from build123d import *
from build123d.topology import SkipClean

# Parameters (mm, degrees)
SKETCH_1_R          = 4
EXTRUDE_1_DEPTH     = 12
SKETCH_3_R          = 15
EXTRUDE_3_DEPTH     = 25
CUT_EXTRUDE_START   = -5
CUT_EXTRUDE_2_DEPTH = 5
SKETCH_6_R          = 4
SKETCH_6_W          = 8
SKETCH_6_H          = 5
CUT_EXTRUDE_3_DEPTH = 69.629439747
SKETCH_10_R         = 7.5
CUT_EXTRUDE_4_DEPTH = 68.037303048


with BuildPart() as part:
    # Sketch 1 → Extrude 1 (new body)
    with BuildSketch(Plane(origin=(0, 0, 0), x_dir=(1, 0, 0), z_dir=(0, 1, 0))):
        with BuildLine():
            ThreePointArc((-40, 25), (-47.071067812, 22.071067812), (-50, 15))
            Line((-50, 15), (-50, -15))
            ThreePointArc((-50, -15), (-47.071067812, -22.071067812), (-40, -25))
            Line((-40, -25), (40, -25))
            ThreePointArc((40, -25), (47.071067812, -22.071067812), (50, -15))
            Line((50, -15), (50, 15))
            ThreePointArc((50, 15), (47.071067812, 22.071067812), (40, 25))
            Line((40, 25), (-40, 25))
        make_face()
        with Locations(Location((-40, -15, 0), (0, 0, 270))):
            Circle(SKETCH_1_R, mode=Mode.SUBTRACT)
        with Locations(Location((40, -15, 0), (0, 0, 270))):
            Circle(SKETCH_1_R, mode=Mode.SUBTRACT)
        with Locations(Location((-40, 15, 0), (0, 0, 270))):
            Circle(SKETCH_1_R, mode=Mode.SUBTRACT)
        with Locations(Location((40, 15, 0), (0, 0, 270))):
            Circle(SKETCH_1_R, mode=Mode.SUBTRACT)
    extrude(amount=EXTRUDE_1_DEPTH)

    # Sketch 3 → Extrude 3 (add)
    with BuildSketch(Plane(origin=(0, 12, 0), x_dir=(1, 0, 0), z_dir=(0, 1, 0))):
        Circle(SKETCH_3_R)
        with BuildLine():
            Line((-50, -4), (-14.456832295, -4))
            ThreePointArc((-14.456832295, -4), (-15, 0), (-14.456832295, 4))
            Line((-14.456832295, 4), (-50, 4))
            Line((-50, 4), (-50, -4))
        make_face()
    extrude_3 = extrude(amount=EXTRUDE_3_DEPTH)

    # Sketch 7 → Cut-Extrude 2 (cut)
    with BuildSketch(Plane(origin=(0, 37, 0), x_dir=(1, 0, 0), z_dir=(0, 1, 0)).offset(CUT_EXTRUDE_START)):
        with BuildLine():
            Line((-14.456832295, 4), (-50, 4))
            Line((-50, 4), (-50, -4))
            Line((-50, -4), (-14.456832295, -4))
            ThreePointArc((-14.456832295, -4), (-15, 0), (-14.456832295, 4))
        make_face()
    cut_extrude_2 = extrude(amount=CUT_EXTRUDE_2_DEPTH, mode=Mode.SUBTRACT)

    # Sketch 6 → Cut-Extrude 3 (cut, symmetric)
    with BuildSketch(Plane.XY.offset(4)):
        with Locations((0.161482291, 22)):
            Circle(SKETCH_6_R)
        Polygon((-14.456832295, 32), (-50, 12), (-50, 32), align=None)
        with Locations((0.271583853, 34.5)):
            Rectangle(SKETCH_6_W, SKETCH_6_H)
    cut_extrude_3 = extrude(amount=CUT_EXTRUDE_3_DEPTH, both=True, mode=Mode.SUBTRACT)

    # Mirror 3: Extrude 3, Cut-Extrude 2, Cut-Extrude 3 across plane
    with SkipClean():  # the faces are left unmerged after this step: merging them gives an invalid solid
        add(extrude_3.mirror(Plane(origin=(0, 0, 0), x_dir=(0, 0, 1), z_dir=(1, 0, 0))))
        add(cut_extrude_2.mirror(Plane(origin=(0, 0, 0), x_dir=(0, 0, 1), z_dir=(1, 0, 0))), mode=Mode.SUBTRACT)
        add(cut_extrude_3.mirror(Plane(origin=(0, 0, 0), x_dir=(0, 0, 1), z_dir=(1, 0, 0))), mode=Mode.SUBTRACT)
    add(part.part.scale(1), mode=Mode.REPLACE)  # the faces are merged on a copy

    # Sketch 10 → Cut-Extrude 4 (cut, through all)
    with BuildSketch(Plane(origin=(0, 37, 0), x_dir=(1, 0, 0), z_dir=(0, 1, 0))):
        with Locations(Location((0, 0, 0), (0, 0, 270))):
            Circle(SKETCH_10_R)
    extrude(amount=-CUT_EXTRUDE_4_DEPTH, mode=Mode.SUBTRACT)


solid = part.part
Read the model definition and answer for the solid it produces. Units are mm, in the model's axes. A direction names the side the tool comes from. Round coordinates to 2 decimals unless told otherwise and drop trailing zeros. Write each loop counter-clockwise with the first axis right and the second up, starting at its lowest first coordinate (ties: lowest second). Pieces come first, ordered by that corner, then holes. Notation, with made-up numbers: (7.25, -14) - (36.25, -14) arc R32 ccw to (36.25, 16) - close; hole circle Ø1 at (-17.75, 52). An arc over 180 degrees is marked (long way). One line per question, with ' | ' between items. Start each with the question number.
1. Section A-A (z = 0) is taken. Determine the outline of the cut face in (x, y).
2. For a pull along X with two mould halves and no side action, classify faces 1 (the face through (31.98, 22.14, -0.06)), 2 (the face through (-12, 0, 0)), 3 (the face through (-50, 6, 0)), 4 (the face through (-4.272, 34, -10)) as +X half, -X half, draft (parallel to the pull), parting line (faces both ways), or undercut.
3. Section D-D (x = 43) is taken. Determine the outline of the cut face in (y, z).
4. For faces 5 (the face through (0, 32, -11)), 6 (the face through (-28, 20, -4)), 7 (the face through (-25, 17, 4)), determine the directions among +Z, -Z, +X, -X, +Y, -Y from which every point of the face is accessible in a straight line to the end or side of a thin tool.
5. Each of these flat-tipped pins is pushed along its axis until it touches: pin 1 (5.5 mm diameter, centred on y = 35, z = 11, fed in from +X); pin 2 (4 mm diameter, centred on y = 33.5, z = -8.5, fed in from +X); pin 3 (1.5 mm diameter, centred on y = 17, z = 0, fed in from -X); pin 4 (1.5 mm diameter, centred on x = -24.5, y = 28, fed in from +Z). Where does it stop, or does it pass through?
6. Section C-C (z = -12) is taken. Determine the outline of the cut face in (x, y), and give its area (3 significant figures).
7. Find the intervals of material crossed by probe 1 along X at (y, z) = (6, 15); probe 2 along Y at (x, z) = (45, 11); probe 3 along X at (y, z) = (22, -11), in increasing order. Write a range as [from, to].
8. Section B-B (y = 22) is taken. Determine the outline of the cut face in (x, z).
Filled in:
1) outline: (-50, 0) - (-7.5, 0) - (-7.5, 37) - (-15, 37) - (-15, 31.69) - (-50, 12) - close; (7.5, 0) - (50, 0) - (50, 12) - (14.46, 32) - (15, 32) - (15, 37) - (7.5, 37) - close
2) face 1: +X half | face 2: draft | face 3: -X half | face 4: undercut
3) outline: (0, -24.54) - (12, -24.54) - (12, -17.65) - (0, -17.65) - close; (0, -12.35) - (12, -12.35) - (12, -4) - (15.94, -4) - (15.94, 4) - (12, 4) - (12, 12.35) - (0, 12.35) - close; (0, 17.65) - (12, 17.65) - (12, 24.54) - (0, 24.54) - close
4) face 5: +Z, -Z, +Y | face 6: -Z, -X, +Y | face 7: +Z, -X, +Y
5) pin 1: x = 12.53 | pin 2: x = 13.52 | pin 3: x = -42.45 | pin 4: through
6) outline: (-50, 0) - (-42.65, 0) - (-42.65, 12) - (-50, 12) - close; (-37.35, 0) - (37.35, 0) - (37.35, 12) - (9, 12) - (9, 37) - (3.73, 37) - (3.73, 32) - (-4.27, 32) - (-4.27, 37) - (-9, 37) - (-9, 12) - (-37.35, 12) - close; (42.65, 0) - (50, 0) - (50, 12) - (42.65, 12) - close; hole circle Ø8 at (-0.16, 22) | area: 1,430 mm²
7) probe 1: [-50, -44], [-36, 36], [44, 50] | probe 2: [0, 12] | probe 3: [-10.2, -4.16], [3.84, 10.2]
8) outline: (-32.23, -4) - (-14.46, -4) arc R15 ccw to (-4.16, -14.41) - (-4.16, -6.24) arc R7.5 cw to (-4.16, 6.24) - (-4.16, 14.41) arc R15 ccw to (-14.46, 4) - (-32.23, 4) - close; (3.84, -14.5) arc R15 ccw to (14.46, -4) - (32.23, -4) - (32.23, 4) - (14.46, 4) arc R15 ccw to (3.84, 14.5) - (3.84, 6.44) arc R7.5 cw to (3.84, -6.44) - close
